Check sheet for the modelled part. Datum: model origin and axes. Units: mm. Face numbers are marked on the shaded views. A direction names the side the tool comes from. Coordinates: 2 decimals unless noted, no trailing zeros. Write each loop counter-clockwise with the first axis right and the second up, starting at its lowest first coordinate (ties: lowest second). Pieces come first, ordered by that corner, then holes. Notation, with made-up numbers: (-9, -23.5) - (27, -23.5) arc R28 cw to (27, -0.5) - close; hole circle Ø3 at (-35.75, 34.25). An arc over 180 degrees is marked (long way). Use one line per item in the form item = value. Start each with the question number.
1. Cross-section at C-C on y = -62. Record the boundary of the cut face in (x, z), then the cut area to 3 significant figures.
2. Draft check along X on the marked faces 3, 4 and 5. Enter one of: +X half, -X half, draft (parallel to the pull), parting line (faces both ways), or undercut.
3. Scan lines: line 1 along Y through (x, z) = (-227, 54.5); line 2 along X through (y, z) = (11, 100.5); line 3 along Z through (x, y) = (44.5, 72). Record each from-to range of solid material in increasing order.
4. Cross-section at B-B on x = -94.5. Record the boundary of the cut face in (y, z), then the cut area to 3 significant figures.
5. Tool access check on the marked faces 1 and 2. Record the directions out of +Z, -Z, +X, -X, +Y, -Y that give a thin tool (end or side, any length) a straight path to the whole face; none if there is none.
6. Cross-section at A-A on z = 96. Record the boundary of the cut face in (x, y).
7. Go/stop test with a flat-tipped pin: pin 1 Ø2 at (x, y) = (-61, 51) entering from +Z. Record where the tip stops, or that it passes through.
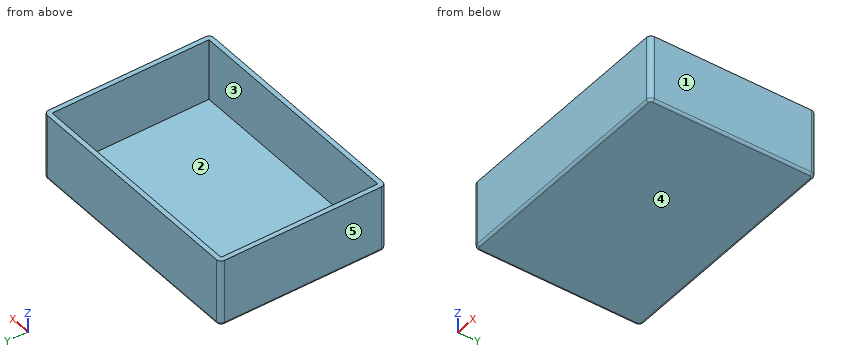
```python
from build123d import *

# Parameters (mm, degrees)
SKETCH1_W           = 500
SKETCH1_H           = 350
BOSS_EXTRUDE2_DEPTH = 140
SKETCH4_W           = 480
SKETCH4_H           = 330
CUT_EXTRUDE3_DEPTH  = 130
FILLET1_R           = 10
FILLET3_R           = 5


with BuildPart() as part:
    # Sketch1 → Boss-Extrude2 (new body)
    with BuildSketch(Plane.XY):
        Rectangle(SKETCH1_W, SKETCH1_H)
    extrude(amount=BOSS_EXTRUDE2_DEPTH)

    # Sketch4 → Cut-Extrude3 (cut)
    with BuildSketch(Plane.XY.offset(140)):
        Rectangle(SKETCH4_W, SKETCH4_H)
    extrude(amount=-CUT_EXTRUDE3_DEPTH, mode=Mode.SUBTRACT)

    # Fillet1
    fillet1_edges = [part.edges().sort_by_distance(p)[0] for p in [
        (250, -175, 70),
        (-250, -175, 70),
        (-250, 175, 70),
        (250, 175, 70),
    ]]
    fillet(fillet1_edges, radius=FILLET1_R)

    # Fillet3
    fillet3_edges = [part.edges().sort_by_distance(p)[0] for p in [
        (0, 175, 0),
        (250, 0, 0),
        (0, -175, 0),
        (-250, 0, 0),
        (-247.071067812, -172.071067812, 0),
        (-247.071067812, 172.071067812, 0),
        (247.071067812, -172.071067812, 0),
        (247.071067812, 172.071067812, 0),
    ]]
    fillet(fillet3_edges, radius=FILLET3_R)


solid = part.part
```
Final values:
q1.outline = (-250, 5) arc R5 ccw to (-245, 0) - (245, 0) arc R5 ccw to (250, 5) - (250, 140) - (240, 140) - (240, 10) - (-240, 10) - (-240, 140) - (-250, 140) - close
q1.area = 7,590 mm²
q2.face_3 = undercut
q2.face_4 = draft
q2.face_5 = -X half
q3.line_1 = -175 to -165, 165 to 175
q3.line_2 = -250 to -240, 240 to 250
q3.line_3 = 0 to 10
q4.outline = (-175, 5) arc R5 ccw to (-170, 0) - (170, 0) arc R5 ccw to (175, 5) - (175, 140) - (165, 140) - (165, 10) - (-165, 10) - (-165, 140) - (-175, 140) - close
q4.area = 6,090 mm²
q5.face_1 = +Z, -Z, +X, +Y, -Y
q5.face_2 = +Z
q6.outline = (-250, -165) arc R10 ccw to (-240, -175) - (240, -175) arc R10 ccw to (250, -165) - (250, 165) arc R10 ccw to (240, 175) - (-240, 175) arc R10 ccw to (-250, 165) - close; hole (-240, -165) - (240, -165) - (240, 165) - (-240, 165) - close
q7.pin_1 = 10
